Design review of the part built by this model. Coordinates are the model's own, in mm. A direction names the side the tool comes from. Coordinates: 2 decimals unless noted, no trailing zeros. Write each loop counter-clockwise with the first axis right and the second up, starting at its lowest first coordinate (ties: lowest second). Pieces come first, ordered by that corner, then holes.
```python
from build123d import *

# Parameters (mm, degrees)
F0_R     = 8.25
F0_R_2   = 6.25
F1_DEPTH = 11
F2_DEPTH = 3
F3_R     = 8.25
F3_R_2   = 1.5
F4_DEPTH = 3
F5_SIZE  = 1


with BuildPart() as f1:
    # F0 (on Top) → F1 (new body)
    with BuildSketch(Plane.XY):
        Circle(F0_R)
        Circle(F0_R_2, mode=Mode.SUBTRACT)
    extrude(amount=F1_DEPTH)

    # F0 (on Top) → F2 (join)
    with BuildSketch(Plane.XY):
        Circle(F0_R)
        Circle(F0_R_2, mode=Mode.SUBTRACT)
        Circle(F0_R_2)
        Polygon((2.9444863729, -1.7), (0, -3.4), (-2.9444863729, -1.7), (-2.9444863729, 1.7), (0, 3.4), (2.9444863729, 1.7), align=None, mode=Mode.SUBTRACT)
    extrude(amount=-F2_DEPTH)

    # F3 (on face) → F4 (join)
    with BuildSketch(Plane(origin=(0, 0, -3), x_dir=(1, 0, 0), z_dir=(0, 0, -1))):
        Circle(F3_R)
        Polygon((0, 3.4), (2.9444863729, 1.7), (2.9444863729, -1.7), (0, -3.4), (-2.9444863729, -1.7), (-2.9444863729, 1.7), align=None, mode=Mode.SUBTRACT)
        Polygon((2.9444863729, -1.7), (2.9444863729, 1.7), (0, 3.4), (-2.9444863729, 1.7), (-2.9444863729, -1.7), (0, -3.4), align=None)
        Circle(F3_R_2, mode=Mode.SUBTRACT)
    extrude(amount=F4_DEPTH)

    # F5
    f5_edges = [f1.edges().sort_by_distance(p)[0] for p in [
        (-8.25, 0, 11),
        (-8.25, 0, -6),
        (-1.5, 0, -6),
    ]]
    chamfer(f5_edges, length=F5_SIZE)


solid = f1.part
```
(1) Consider section C-C (z = 4.25). Give the boundary of the cut face in (x, y), plus the area to 3 significant figures.
(2) Consider section B-B (z = -1.75). Give the boundary of the cut face in (x, y), plus the area to 3 significant figures.
(3) Insertion check: pin 1 Ø1 at (x, z) = (-4, -1.5) entering from +Y; pin 2 Ø1.8 at (x, y) = (-0.5, 1.5) entering from +Z; pin 3 Ø1.5 at (y, z) = (0.5, -1.5) entering from -X. Each pin has a flat end and moves straight along its axis. Give the tip position at first contact, or say it passes through.
(4) Mouldability with a two-part tool opening along X and no side actions: class faces 1 (the flat face through (3, 0, -6)), 2 (the cylindrical face through (5.96, 1.88, 5.42)) as +X half, -X half, draft (parallel to the pull), parting line (faces both ways), or undercut.
(5) For faces 3 (the flat face through (1.49, -2.54, -1.48)), 4 (the flat face through (0, 6.5, 11)), list the 3-axis set-ups (+Z, -Z, +X, -X, +Y, -Y) from which the entire face can be reached by the end or side of a thin tool; tool diameter is ignored.
(6) Wall thickness on line 1 (Y direction, x = 0, z = -4.1); line 2 (Y direction, x = 0, z = 5): over which ranges is each line inside the solid? List them lowest first.
(7) Consider section A-A (y = 0). Give the boundary of the cut face in (x, z).
Results:
1. outline: circle Ø16.5 at (0, 0); hole circle Ø12.5 at (0, 0)
1. area: 91.1 mm2
2. outline: circle Ø16.5 at (0, 0); hole (-2.94, -1.7) - (0, -3.4) - (2.94, -1.7) - (2.94, 1.7) - (0, 3.4) - (-2.94, 1.7) - close
2. area: 184 mm2
3. pin 1: stops at y = 7.47
3. pin 2: stops at z = -3
3. pin 3: stops at x = -8.25
4. face 1: draft
4. face 2: undercut
5. face 3: +Z
5. face 4: +Z, +X, -X, +Y, -Y
6. line 1: y = -8.25 to -1.5, 1.5 to 8.25
6. line 2: y = -8.25 to -6.25, 6.25 to 8.25
7. outline: (-8.25, -5) - (-7.25, -6) - (-2.5, -6) - (-1.5, -5) - (-1.5, -3) - (-2.94, -3) - (-2.94, 0) - (-6.25, 0) - (-6.25, 11) - (-7.25, 11) - (-8.25, 10) - close; (1.5, -5) - (2.5, -6) - (7.25, -6) - (8.25, -5) - (8.25, 10) - (7.25, 11) - (6.25, 11) - (6.25, 0) - (2.94, 0) - (2.94, -3) - (1.5, -3) - close
